Check sheet for the drawn part. Datum: minimum x, y, z corner. Units: mm. Give positions to 0.01 mm unless a question says otherwise; leave off trailing zeros. Loops run counter-clockwise (first coordinate to the right, second up) from the corner with the lowest first, then second, coordinate; pieces in that order, holes last. Notation, with made-up numbers: (1.5, 48) -> (9.5, 48) arc R30 ccw to (9.5, 80) -> close; hole circle Ø6 at (0.25, -17). An arc over 180 degrees is marked (long way). One line per question, with ' | ' between items.
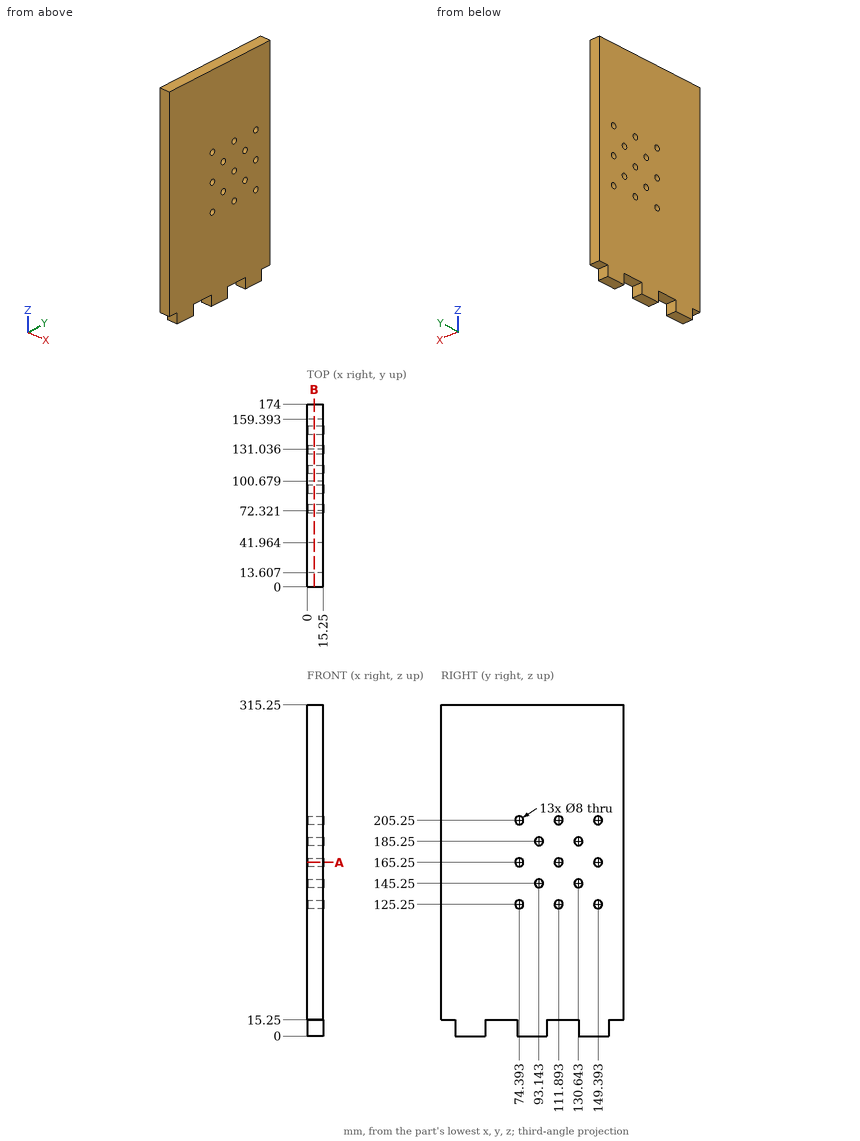
Item 1: Sectioned sample at B-B (x = 6.75). Give the number of separate pieces and of enclosed holes in the cut face, plus the area to 3 significant figures.
Result:
separate pieces: 1 | enclosed holes: 13 | area: 52,800 mm2
Item 2: Sectioned sample at A-A (z = 165.25). Record the cut outline in (x, y).
Result:
outline: (0, 0) -> (15.25, 0) -> (15.25, 70.39) -> (0, 70.39) -> close; (0, 78.39) -> (15.25, 78.39) -> (15.25, 107.89) -> (0, 107.89) -> close; (0, 115.89) -> (15.25, 115.89) -> (15.25, 145.39) -> (0, 145.39) -> close; (0, 153.39) -> (15.25, 153.39) -> (15.25, 174) -> (0, 174) -> close
Item 3: Scan lines: probe 1 along Y at (x, z) = (10.5, 165.25); probe 2 along Y at (x, z) = (13.25, 126); probe 3 along Y at (x, z) = (8.75, 185.25). Record each from-to range of solid material in increasing order.
Result:
probe 1: 0 to 70.39, 78.39 to 107.89, 115.89 to 145.39, 153.39 to 174 | probe 2: 0 to 70.46, 78.32 to 107.96, 115.82 to 145.46, 153.32 to 174 | probe 3: 0 to 89.14, 97.14 to 126.64, 134.64 to 174
Item 4: Depth check by flat-ended pin: pin 1 Ø7 at (y, z) = (74.39, 165.25) entering from -X; pin 2 Ø4.5 at (x, z) = (5.5, 10.5) entering from -Y. Enter the tip coordinate at first touch or a pass-through.
Result:
pin 1: through | pin 2: y = 13.61
